Can you work these out from the model? Positions are in its coordinate system, mm. A direction names the side the tool comes from. Give positions to 0.01 mm unless a question says otherwise; leave off trailing zeros.
from build123d import *

# Parameters (mm, degrees)
F0_W     = 2
F0_H     = 8
F3_DEPTH = 25


with BuildPart() as f1:
    # F0 (on Front) → F1 (revolve)
    with BuildSketch(Plane.XZ):
        with BuildLine():
            Line((-53.7507587761, 0), (-16, 0))
            Line((-16, 0), (-16, 8))
            Line((-16, 8), (-45.5, 8))
            Line((-45.5, 8), (-59.45, 4.3))
            Line((-59.45, 4.3), (-59.45, 0))
            Line((-59.45, 0), (-56.548682875, 0))
            ThreePointArc((-56.548682875, 0), (-56.4072615188, 0.0585786438), (-56.348682875, 0.2))
            Line((-56.348682875, 0.2), (-56.348682875, 0.3437917702))
            ThreePointArc((-56.348682875, 0.3437917702), (-56.35, 0.4), (-56.348682875, 0.4562082298))
            ThreePointArc((-56.348682875, 0.4562082298), (-55.1432237144, 1.5999808673), (-53.9507587761, 0.442667165))
            ThreePointArc((-53.9507587761, 0.442667165), (-53.95, 0.4), (-53.9507587761, 0.357332835))
            Line((-53.9507587761, 0.357332835), (-53.9507587761, 0.2))
            ThreePointArc((-53.9507587761, 0.2), (-53.8921801324, 0.0585786438), (-53.7507587761, 0))
        make_face()
        with Locations((-13, 4)):
            Rectangle(F0_W, F0_H)
        with Locations((-15, 4)):
            Rectangle(F0_W, F0_H)
        Polygon((-12, 0), (-8.5, 0), (-8.5, 3.2), (-10.5, 3.2), (-10.5, 8), (-12, 8), align=None)
    revolve(axis=Axis((0, 0, 5.6), (0, 0, -1)))

    # F2 (on face) → F3 (cut)
    with BuildSketch(Plane.XY.offset(8)):
        with BuildLine():
            ThreePointArc((-13.8571428571, -1.9948914348), (-14, 0), (-13.8571428571, 1.9948914348))
            ThreePointArc((-13.8571428571, 1.9948914348), (-16, 0), (-13.8571428571, -1.9948914348))
        make_face()
        with BuildLine():
            ThreePointArc((-12, 0), (-12.5361498906, 1.3627702877), (-13.8571428571, 1.9948914348))
            ThreePointArc((-13.8571428571, 1.9948914348), (-14, 0), (-13.8571428571, -1.9948914348))
            ThreePointArc((-13.8571428571, -1.9948914348), (-12.5361498906, -1.3627702877), (-12, 0))
        make_face()
        with BuildLine():
            ThreePointArc((13.8571428571, -1.9948914348), (13.9642400438, -1), (14, 0))
            ThreePointArc((14, 0), (13.9642400438, 1), (13.8571428571, 1.9948914348))
            ThreePointArc((13.8571428571, 1.9948914348), (12, 0), (13.8571428571, -1.9948914348))
        make_face()
        with BuildLine():
            ThreePointArc((13.8571428571, 1.9948914348), (13.9642400438, 1), (14, 0))
            ThreePointArc((14, 0), (13.9642400438, -1), (13.8571428571, -1.9948914348))
            ThreePointArc((13.8571428571, -1.9948914348), (15.3627702877, -1.4638501094), (16, 0))
            ThreePointArc((16, 0), (15.3627702877, 1.4638501094), (13.8571428571, 1.9948914348))
        make_face()
    extrude(amount=-F3_DEPTH, mode=Mode.SUBTRACT)


solid = f1.part
(1) Will these pins go through, and if not, where does the flat tip stop? P1, Ø10.5, axis at x = -0.5, y = -2, coming from the +Z side; P2, Ø19, axis at x = 0, y = 0, coming from the +Z side; P3, Ø2, axis at x = -20.5, z = 3.5, coming from the -Y side; P4, Ø1.5, axis at y = 30.5, z = 4, coming from the +X side.
Returned:
P1: passes through
P2: stops at z = 3.2
P3: stops at y = -56.16
P4: stops at x = 51.47
(2) Please list where these lines run through material, in increasing order: probe 1 along Y at (x, z) = (-44, 1); probe 2 along Z at (x, y) = (-7, 6); probe 3 along Y at (x, z) = (-7, 3.5).
Returned:
probe 1: y = -39.98 to -34.95, -31.5 to 31.5, 34.95 to 39.98
probe 2: z = 0 to 3.2
probe 3: y = -59.04 to -7.83, 7.83 to 59.04
(3) Thinking about a two-plate mould opening in Y: for faces 3 (the conical face through (10.05, -45.27, 7.77)), 4 (the flat face through (-11, 1, 0)), 5 (the cylindrical face through (-4.57, 7.167, 1.622)), 6 (the cylindrical face through (-10, 3.2, 5.6)), which applies, pulls with the +Y half, pulls with the -Y half, needs draft (parallel to the pull), parting line crosses it, or undercut?
Returned:
face 3: parting line crosses it
face 4: needs draft
face 5: undercut
face 6: undercut
(4) Which directions (+Z, -Z, +X, -X, +Y, -Y) give clear straight access to the entire face, cutting with the end or side of a thin tool? Please do faces 1 (the flat face through (9, 0, 3.2)), 2 (the cylindrical face through (47.18, -36.17, 2.12)).
Returned:
face 1: +Z
face 2: +Z, -Z
